Read the model definition and answer for the solid it produces. Units are mm, in the model's axes. Face numbers are marked on the shaded views. Give positions to 0.01 mm unless a question says otherwise; leave off trailing zeros. Order: outer loops, then holes, each group sorted by start corner. A loop starts at its lowest first (then second) coordinate and runs counter-clockwise, first axis right, second up. Notation, with made-up numbers: M -8.5,81 L 30.5,81 A20 cw 30.5,108 Z; hole C 37.5,-36 d3. An arc over 180 degrees is marked long. One line per item, written item: value. Start each with the question number.
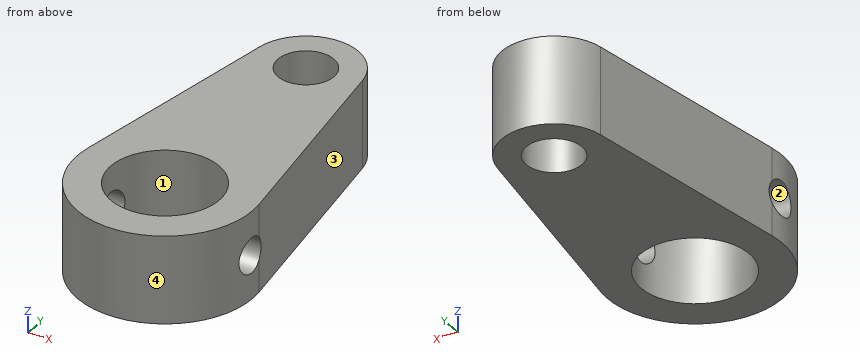
from build123d import *

# Parameters (mm, degrees)
CROQUIS1_R                 = 3.1
CROQUIS1_R_2               = 1.6
SALIENTE_EXTRUIR1_DEPTH    = 5
CORTAR_EXTRUIR1_DEPTH      = 18.33749982
CORTAR_EXTRUIR1_DEPTH_BACK = 18.33749982
CROQUIS3_R                 = 1


with BuildPart() as part:
    # Croquis1 → Saliente-Extruir1 (new body)
    with BuildSketch(Plane.XY):
        with BuildLine():
            Line((-4.938876333, 0.779423227), (-2.9633258, 13.297653936))
            ThreePointArc((-2.9633258, 13.297653936), (0, 15.83), (2.9633258, 13.297653936))
            Line((2.9633258, 13.297653936), (4.938876333, 0.779423227))
            ThreePointArc((4.938876333, 0.779423227), (0, -5), (-4.938876333, 0.779423227))
        make_face()
        Circle(CROQUIS1_R, mode=Mode.SUBTRACT)
        with Locations((0, 12.83)):
            Circle(CROQUIS1_R_2, mode=Mode.SUBTRACT)
    extrude(amount=SALIENTE_EXTRUIR1_DEPTH)

    # Croquis3 → Cortar-Extruir1 (cut, two sides: drawn at the far end of the back side and taken through both)
    with BuildSketch(Plane(origin=(0, 0, 0), x_dir=(0, 0, -1), z_dir=(1, 0, 0)).offset(-CORTAR_EXTRUIR1_DEPTH_BACK)):
        with Locations((-2.5, 0)):
            Circle(CROQUIS3_R)
    extrude(amount=CORTAR_EXTRUIR1_DEPTH + CORTAR_EXTRUIR1_DEPTH_BACK, mode=Mode.SUBTRACT)


solid = part.part
Q1. Find section C-C, the plane x = 0. Give the vertices of the cut face in (y, z).
Q2. Determine the mould class of the marked faces 1, 2, 3 and 4 for opening direction X: released by +X, released by -X, zero draft, split by the parting line, or undercut.
Q3. Find section B-B, the plane y = 0. Give the vertices of the cut face in (x, z).
Q4. Each of these flat-tipped pins is pushed along its axis until it touches: pin 1 (3 mm diameter, centred on x = 2, y = 13.5, fed in from -Z); pin 2 (2 mm diameter, centred on y = 13, z = 1, fed in from -X). Where does it stop, or does it pass through?
Q5. Find section A-A, the plane z = 2.5. Give the vertices of the cut face in (x, y).
Q6. Consider probe 1 along Y at (x, z) = (-1, 1.45); probe 2 along Y at (x, z) = (-0.5, 2.9); probe 3 along Z at (x, y) = (4, 0). Determine where each line is inside the solid, lowest interval first.
Q7. Find section D-D, the plane z = 3.75. Give the vertices of the cut face in (x, y).
Evaluation:
1. outline: M -5,0 L -3.1,0 L -3.1,5 L -5,5 Z; M 3.1,0 L 11.23,0 L 11.23,5 L 3.1,5 Z; M 14.43,0 L 15.83,0 L 15.83,5 L 14.43,5 Z
2. face 1: undercut
2. face 2: zero draft
2. face 3: released by +X
2. face 4: split by the parting line
3. outline: M -5,0 L -3.1,0 L -3.1,1.5 L -5,1.5 Z; M -5,3.5 L -3.1,3.5 L -3.1,5 L -5,5 Z; M 3.1,0 L 5,0 L 5,1.5 L 3.1,1.5 Z; M 3.1,3.5 L 5,3.5 L 5,5 L 3.1,5 Z
4. pin 1: z = 0
4. pin 2: x = -3.17
5. outline: M -4.9,-1 A5 ccw 4.9,-1 L 2.93,-1 A3.1 cw -2.93,-1 Z; M -4.9,1 L -2.93,1 A3.1 cw 2.93,1 L 4.9,1 L 2.96,13.3 A3 ccw -2.96,13.3 Z; hole C 0,12.83 d3.2
6. probe 1: -4.9 to -2.93, 2.93 to 11.58, 14.08 to 15.66
6. probe 2: -4.97 to -3.06, 3.06 to 11.31, 14.35 to 15.79
6. probe 3: 0 to 1.5, 3.5 to 5
7. outline: M -4.94,0.78 A5 ccw long 4.94,0.78 L 2.96,13.3 A3 ccw -2.96,13.3 Z; hole C 0,0 d6.2; hole C 0,12.83 d3.2
